Geometry check sheet. Reference: drawing and pictorial views, mm from the part's lowest x, y, z. Coordinates: 2 decimals unless noted, no trailing zeros. Write each loop counter-clockwise with the first axis right and the second up, starting at its lowest first coordinate (ties: lowest second). Pieces come first, ordered by that corner, then holes. Notation, with made-up numbers: M 82.25,-33.75 L 130.25,-33.75 A26 cw 130.25,-11.75 Z; hole C -27,70.5 d10. An arc over 180 degrees is marked long. One line per item, written item: value.
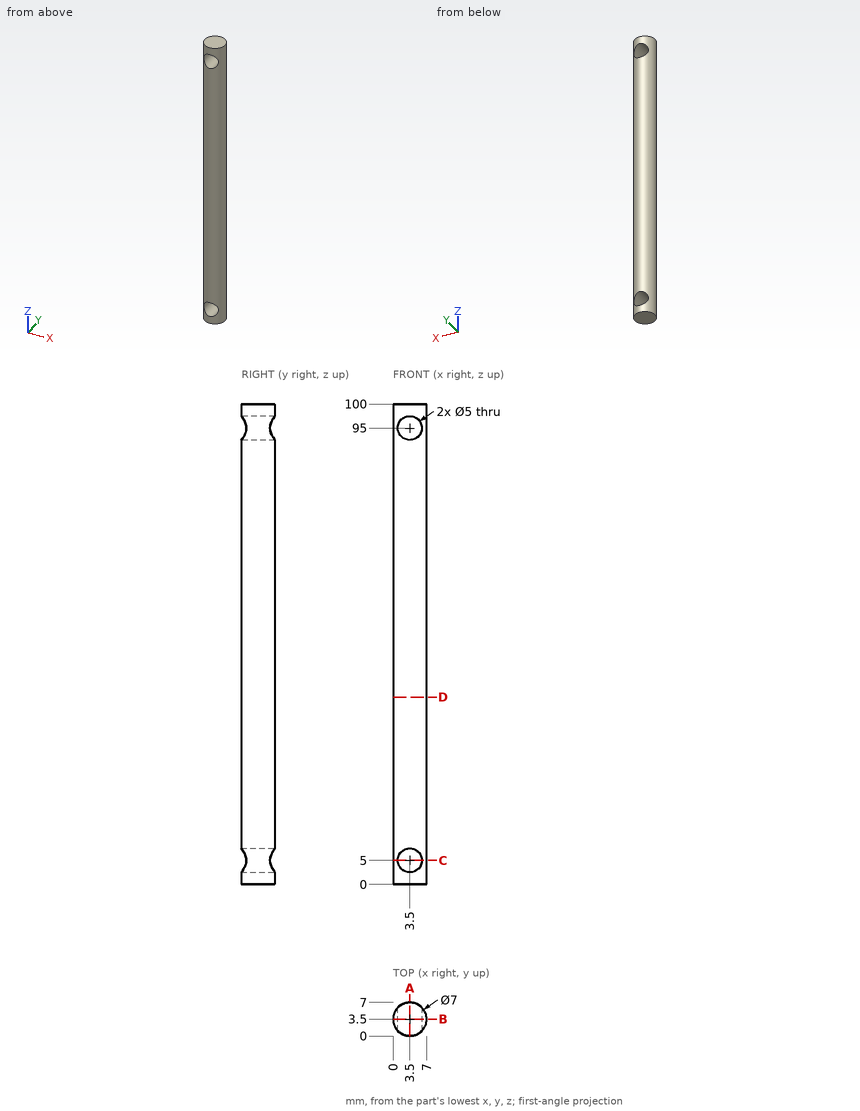
Item 1: Scan lines: line 1 (Z direction, x = 3.5, y = 4); line 2 (Z direction, x = 3, y = 2.5); line 3 (X direction, y = 5.25, z = 70.5). Record each from-to range of solid material in increasing order.
The answers:
line 1: z = 0 to 2.5, 7.5 to 92.5, 97.5 to 100
line 2: z = 0 to 2.55, 7.45 to 92.55, 97.45 to 100
line 3: x = 0.47 to 6.53
Item 2: Cross-section at D-D, the plane z = 39. Enter the section's corners in (x, y), and give its area (3 significant figures).
The answers:
outline: C 3.5,3.5 d7
area: 38.5 mm²
Item 3: Cross-section at A-A, the plane x = 3.5. Enter the section's corners in (y, z).
The answers:
outline: M 0,0 L 7,0 L 7,2.5 L 0,2.5 Z; M 0,7.5 L 7,7.5 L 7,92.5 L 0,92.5 Z; M 0,97.5 L 7,97.5 L 7,100 L 0,100 Z
Item 4: Go/stop test with flat-tipped pins: P1, Ø2, axis at x = 1, z = 79, coming from the -Y side; P2, Ø1, axis at x = 4, z = 70, coming from the +Y side. Record where each tip stops, or that it passes through.
The answers:
P1: stops at y = 0.34
P2: stops at y = 7
Item 5: Cross-section at B-B, the plane y = 3.5. Enter the section's corners in (x, z), and give its area (3 significant figures).
The answers:
outline: M 0,0 L 7,0 L 7,100 L 0,100 Z; hole C 3.5,5 d5; hole C 3.5,95 d5
area: 661 mm²
Item 6: Cross-section at C-C, the plane z = 5. Enter the section's corners in (x, y).
The answers:
outline: M 1,1.05 L 1,5.95 A3.5 ccw Z; M 6,1.05 A3.5 ccw 6,5.95 Z
